Input: part model. Units: mm. Frame: model coordinates. A direction names the side the tool comes from. Give positions to 0.01 mm unless a question says otherwise; leave off trailing zeros. Loops run counter-clockwise (first coordinate to the right, second up) from the corner with the lowest first, then second, coordinate; pieces in that order, holes last. Notation, with made-up numbers: M -9,29 L 42,29 A8 ccw 42,34 Z; hole C 39.25,28.5 d9. An arc over 180 degrees is marked long. One line per item, written item: value. Start each with the question number.
(1) Section A-A on z = 1.75. Output: boundary loops of the cut face in (x, y), plus the area to 3 significant figures.
(2) Pull-direction query (X, two-part tool) for faces 1 (the cylindrical face through (-10, 10, 0)), 2 (the cylindrical face through (604.619, 8.085, -0.14)), 3 (the flat face through (310, -25, 0)); classes: released by +X, released by -X, zero draft, split by the parting line, or undercut.
(3) Section B-B on x = 85.5. Output: boundary loops of the cut face in (y, z), plus the area to 3 significant figures.
(4) Access query for faces 4 (the flat face through (453, 0, 0)), 5 (the flat face through (299, 7, 10)), 6 (the flat face through (143, 0, 0)). Directions: +Z, -Z, +X, -X, +Y, -Y. A direction counts if a zero-diameter tool reaches every point of the face in a straight line with its end or side. Return the directions, or none.
(5) Ray query, line 1 along Y through (x, z) = (0, -5); line 2 along X through (y, z) = (-13.5, 4); line 3 along X through (y, z) = (-50.5, -6.75). Return the intervals inside material, ascending. Write a range as from..to.
(6) Section C-C on y = -15. Output: boundary loops of the cut face in (x, z), plus the area to 3 significant figures.
(7) Pin query (flat end, axial travel): P1, Ø1, axis at y = 11.5, z = 5.5, coming from the -X side; P2, Ø1.5, axis at x = 303.5, z = 7, coming from the -Y side; P3, Ø6, axis at x = 114, z = 6.5, coming from the -Y side. Return the tip coordinate at first contact, or that it passes through.
```python
from build123d import *

# Parameters (mm, degrees)
F0_R     = 5
F1_DEPTH = 10


with BuildPart() as f1:
    # F0 (on Top) → F1 (new body, symmetric)
    with BuildSketch(Plane.XY):
        with BuildLine():
            ThreePointArc((0, 20), (-10, 10), (0, 0))
            Line((0, 0), (290, 0))
            Line((290, 0), (290, -50))
            ThreePointArc((290, -50), (300, -60), (310, -50))
            Line((310, -50), (310, 0))
            Line((310, 0), (600, 0))
            ThreePointArc((600, 0), (610, 10), (600, 20))
            Line((600, 20), (0, 20))
        make_face()
        with Locations((300, -50)):
            Circle(F0_R, mode=Mode.SUBTRACT)
        with Locations((0, 10)):
            Circle(F0_R, mode=Mode.SUBTRACT)
        with Locations((600, 10)):
            Circle(F0_R, mode=Mode.SUBTRACT)
    extrude(amount=F1_DEPTH, both=True)


solid = f1.part
```
Output values:
1. outline: M 0,0 L 290,0 L 290,-50 A10 ccw 310,-50 L 310,0 L 600,0 A10 ccw 600,20 L 0,20 A10 ccw Z; hole C 0,10 d10; hole C 300,-50 d10; hole C 600,10 d10
1. area: 13,200 mm²
2. face 1: released by -X
2. face 2: undercut
2. face 3: released by +X
3. outline: M 0,-10 L 20,-10 L 20,10 L 0,10 Z
3. area: 400 mm²
4. face 4: +Z, -Z, +X, -Y
4. face 5: +Z, +X, -X, +Y, -Y
4. face 6: +Z, -Z, -X, -Y
5. line 1: y = 0..5, 15..20
5. line 2: x = 290..310
5. line 3: x = 290.01..295.03, 304.97..309.99
6. outline: M 290,-10 L 310,-10 L 310,10 L 290,10 Z
6. area: 400 mm²
7. P1: stops at x = -9.95
7. P2: stops at y = -59.61
7. P3: stops at y = 0
